Part model, mm, in its own coordinate system. Round coordinates to 2 decimals unless told otherwise and drop trailing zeros. Write each loop counter-clockwise with the first axis right and the second up, starting at its lowest first coordinate (ties: lowest second). Pieces come first, ordered by that corner, then holes. Notation, with made-up numbers: M -5.5,-0.75 L 51.5,-0.75 A24 cw 51.5,15.25 Z; hole C 12.5,83.5 d6. An arc over 180 degrees is marked long. Use one line per item in the form item = value. Start each with the question number.
Item 1: Cut at D-D, the plane z = 217. Give the cut face in (x, y).
Item 2: Flat gauge pins, fed straight in: pin 1 Ø1 at (x, y) = (4, 62.5) entering from -Z; pin 2 Ø1.5 at (x, z) = (3.5, 78.5) entering from -Y. Where does each tip first touch, or does it go through?
Item 3: Probe L1, parallel to Z at x = 4.3, y = 85; L2, parallel to Z at x = 3.4, y = 251; L3, parallel to Y at x = 3.3, z = 223. List the from-to ranges inside material, lowest first.
Item 4: Cut at A-A, the plane y = 115. Give the cut face in (x, z).
Item 5: Cut at B-B, the plane y = -2.5. Give the cut face in (x, z), then the cut area to 3 significant figures.
Item 6: Cut at C-C, the plane x = 0.9. State how many separate pieces and enclosed holes the cut face has, then the cut area to 3 significant figures.
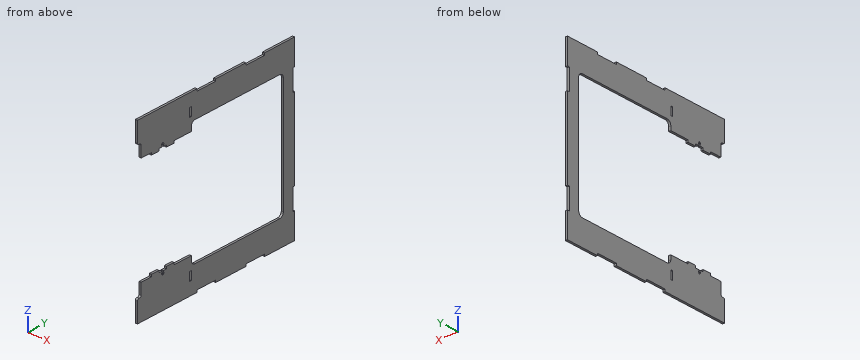
from build123d import *

# Parameters (mm, degrees)
SKETCH_1_W      = 20
SKETCH_1_H      = 5
EXTRUDE_1_DEPTH = 5


with BuildPart() as part:
    # 草图1 → 凸台-拉伸1 (new body)
    with BuildSketch(Plane(origin=(0, 0, 0), x_dir=(0, 0, -1), z_dir=(1, 0, 0))):
        with BuildLine():
            Line((-80, 27), (-80, -19))
            Line((-80, -19), (-85, -19))
            Line((-85, -19), (-85, -39))
            Line((-85, -39), (-80, -39))
            Line((-80, -39), (-80, -47.5))
            Line((-80, -47.5), (-77, -47.5))
            Line((-77, -47.5), (-77, -46.25))
            Line((-77, -46.25), (-74, -46.25))
            Line((-74, -46.25), (-74, -47.5))
            Line((-74, -47.5), (-72, -47.5))
            Line((-72, -47.5), (-72, -50.5))
            Line((-72, -50.5), (-74, -50.5))
            Line((-74, -50.5), (-74, -51.75))
            Line((-74, -51.75), (-77, -51.75))
            Line((-77, -51.75), (-77, -50.5))
            Line((-77, -50.5), (-80, -50.5))
            Line((-80, -50.5), (-80, -59))
            Line((-80, -59), (-85, -59))
            Line((-85, -59), (-85, -79))
            Line((-85, -79), (-80, -79))
            Line((-80, -79), (-80, -90.3))
            Line((-80, -90.3), (-80, -106.3))
            Line((-80, -106.3), (-54, -106.3))
            ThreePointArc((-54, -106.3), (-51.171572875, -107.471572875), (-50, -110.3))
            Line((-50, -110.3), (-50, -112.3))
            ThreePointArc((-50, -112.3), (-48.828427125, -115.128427125), (-46, -116.3))
            Line((-46, -116.3), (0, -116.3))
            Line((0, -116.3), (0, -64.3))
            Line((0, -64.3), (0, 0))
            Line((0, 0), (0, 42))
            Line((0, 42), (-5, 42))
            Line((-5, 42), (-5, 92))
            Line((-5, 92), (0, 92))
            Line((0, 92), (0, 172))
            Line((0, 172), (-5, 172))
            Line((-5, 172), (-5, 222))
            Line((-5, 222), (0, 222))
            Line((0, 222), (0, 302))
            Line((0, 302), (-60, 302))
            Line((-60, 302), (-60, 297))
            Line((-60, 297), (-110, 297))
            Line((-110, 297), (-110, 302))
            Line((-110, 302), (-300, 302))
            Line((-300, 302), (-300, 297))
            Line((-300, 297), (-350, 297))
            Line((-350, 297), (-350, 302))
            Line((-350, 302), (-410, 302))
            Line((-410, 302), (-410, 222))
            Line((-410, 222), (-405, 222))
            Line((-405, 222), (-405, 172))
            Line((-405, 172), (-410, 172))
            Line((-410, 172), (-410, 92))
            Line((-410, 92), (-405, 92))
            Line((-405, 92), (-405, 42))
            Line((-405, 42), (-410, 42))
            Line((-410, 42), (-410, -90.3))
            Line((-410, -90.3), (-410, -116.3))
            Line((-410, -116.3), (-364, -116.3))
            ThreePointArc((-364, -116.3), (-361.171572875, -115.128427125), (-360, -112.3))
            Line((-360, -112.3), (-360, -110.3))
            ThreePointArc((-360, -110.3), (-358.828427125, -107.471572875), (-356, -106.3))
            Line((-356, -106.3), (-330, -106.3))
            Line((-330, -106.3), (-330, -90.3))
            Line((-330, -90.3), (-330, -79))
            Line((-330, -79), (-325, -79))
            Line((-325, -79), (-325, -59))
            Line((-325, -59), (-330, -59))
            Line((-330, -59), (-330, -50.5))
            Line((-330, -50.5), (-333, -50.5))
            Line((-333, -50.5), (-333, -51.75))
            Line((-333, -51.75), (-336, -51.75))
            Line((-336, -51.75), (-336, -50.5))
            Line((-336, -50.5), (-338, -50.5))
            Line((-338, -50.5), (-338, -47.5))
            Line((-338, -47.5), (-336, -47.5))
            Line((-336, -47.5), (-336, -46.25))
            Line((-336, -46.25), (-333, -46.25))
            Line((-333, -46.25), (-333, -47.5))
            Line((-333, -47.5), (-330, -47.5))
            Line((-330, -47.5), (-330, -39))
            Line((-330, -39), (-325, -39))
            Line((-325, -39), (-325, -19))
            Line((-325, -19), (-330, -19))
            Line((-330, -19), (-330, 27))
            Line((-330, 27), (-340, 27))
            ThreePointArc((-340, 27), (-347.071067812, 29.928932188), (-350, 37))
            Line((-350, 37), (-350, 262))
            ThreePointArc((-350, 262), (-347.071067812, 269.071067812), (-340, 272))
            Line((-340, 272), (-70, 272))
            ThreePointArc((-70, 272), (-62.928932188, 269.071067812), (-60, 262))
            Line((-60, 262), (-60, 37))
            ThreePointArc((-60, 37), (-62.928932188, 29.928932188), (-70, 27))
            Line((-70, 27), (-80, 27))
        make_face()
        with Locations((-40, 24.5)):
            Rectangle(SKETCH_1_W, SKETCH_1_H, mode=Mode.SUBTRACT)
        with Locations((-370, 24.5)):
            Rectangle(SKETCH_1_W, SKETCH_1_H, mode=Mode.SUBTRACT)
    extrude(amount=EXTRUDE_1_DEPTH)


solid = part.part
Model answer:
q1.outline = M 0,272 L 5,272 L 5,302 L 0,302 Z
q2.pin_1 = 5
q2.pin_2 = -106.3
q3.L1 = 5 to 60, 350 to 405
q3.L2 = 0 to 60, 350 to 410
q3.L3 = 272 to 302
q4.outline = M 0,0 L 5,0 L 5,60 L 0,60 Z; M 0,350 L 5,350 L 5,410 L 0,410 Z
q5.outline = M 0,0 L 5,0 L 5,80 L 0,80 Z; M 0,330 L 5,330 L 5,410 L 0,410 Z
q5.area = 800 mm²
q6.separate_pieces = 1
q6.enclosed_holes = 2
q6.area = 62,800 mm²
